Check sheet for the modelled part. Datum: model origin and axes. Units: mm. A direction names the side the tool comes from. Give positions to 0.01 mm unless a question says otherwise; leave off trailing zeros. Order: outer loops, then holes, each group sorted by start corner. A loop starts at its lowest first (then second) coordinate and runs counter-clockwise, first axis right, second up.
```python
from build123d import *

# Parameters (mm, degrees)
EXTRUDE_THIN1_DEPTH = 5
SKETCH2_R           = 2
CUT_EXTRUDE1_DEPTH  = 3
FILLET1_R           = 5
FILLET2_R           = 3
FILLET3_R           = 3
FILLET5_R           = 5


with BuildPart() as part:
    # Sketch1 → Extrude-Thin1 (new body)
    with BuildSketch(Plane.XY):
        with BuildLine():
            ThreePointArc((0, 0), (1.709468812, -15.258106238), (6, -30))
            Line((6, -30), (30, -30))
            Line((30, -30), (30, -40))
            Line((30, -40), (-0.59396654, -40))
            ThreePointArc((-0.59396654, -40), (-7.355075067, -20.616040357), (-9.996685535, -0.257445757))
            Line((-9.996685535, -0.257445757), (0, 0))
        make_face()
    extrude(amount=EXTRUDE_THIN1_DEPTH)

    # Sketch2 → Cut-Extrude1 (cut)
    with BuildSketch(Plane(origin=(0, 0, 0), x_dir=(1, 0, 0), z_dir=(0, 1, 0))):
        with Locations(Location((-4.998342767, -2.5, 0), (0, 0, 270))):
            Circle(SKETCH2_R)
    extrude(amount=-CUT_EXTRUDE1_DEPTH, mode=Mode.SUBTRACT)

    # Fillet1
    fillet1_edges = [part.edges().sort_by_distance(p)[0] for p in [
        (30, -30, 2.5),
    ]]
    fillet(fillet1_edges, radius=FILLET1_R)

    # Fillet2
    fillet2_edges = [part.edges().sort_by_distance(p)[0] for p in [
        (30, -40, 2.5),
    ]]
    fillet(fillet2_edges, radius=FILLET2_R)

    # Fillet3
    fillet3_edges = [part.edges().sort_by_distance(p)[0] for p in [
        (6, -30, 2.5),
    ]]
    fillet(fillet3_edges, radius=FILLET3_R)

    # Fillet4
    # a fillet whose section is not a circle: 5, 0.4 mm, written as the material it takes off along each edge (its section moved 0.00015 mm through the faces so that the kernel can cut it)
    with BuildSketch(Plane(origin=(-22.492542459, -0.579252954, 0), x_dir=(0.02574457573397758, -0.9996685530315923, -2.999999998649999e-05), z_dir=(0.9996685534814432, 0.025744575745562638, 0))) as fillet4_piece_1:
        with BuildLine():
            Bezier((5.000000002, 0), (-0.000149995, 0.000150004), (-0.000162, -0.399999995), weights=[1, 0.707106781, 1])
            Line((-0.000162, -0.399999995), (-0.100162, -0.399996995))
            ThreePointArc((-0.100162, -0.399996995), (-0.100006, -0.199997), (-0.1, 3e-06))
            Line((-0.1, 3e-06), (3e-06, 0.1))
            ThreePointArc((3e-06, 0.1), (2.500002999, 0.099925), (5.000003002, 0.1))
            Line((5.000003002, 0.1), (5.000000002, 0))
        make_face()
    extrude(amount=35.000000011, mode=Mode.SUBTRACT)
    with BuildSketch(Plane(origin=(-9.996685535, -0.257445757, -12.554427483), x_dir=(0.9996611732267645, 0.026029574389313356, 0), z_dir=(0, 0, 1))) as fillet4_piece_2:
        with BuildLine():
            Bezier((0.526141916, 0), (-0.126969786, 0.000186198), (0.12506971, -5.02021329), weights=[1, 0.689048379, 1])
            Line((0.12506971, -5.02021329), (0.02519549, -5.025227283))
            ThreePointArc((0.02519549, -5.025227283), (-0.069016975, -2.513387959), (-0.099999996, 2.8509e-05))
            Line((-0.099999996, 2.8509e-05), (2.8509e-05, 0.099999996))
            ThreePointArc((2.8509e-05, 0.099999996), (0.263099446, 0.099924996), (0.526170426, 0.099999996))
            Line((0.526170426, 0.099999996), (0.526141916, 0))
        make_face()
    extrude(amount=30.108854967, mode=Mode.SUBTRACT)
    with BuildSketch(Plane(origin=(-22.492542459, -0.579252954, 5), x_dir=(-9.654215225776052e-06, 0.00037487568119717526, -0.9999999296875075), z_dir=(0.9996685534814432, 0.025744575745562638, 0))) as fillet4_piece_3:
        with BuildLine():
            Bezier((0.400000028, 0), (-0.000149944, 0.000150056), (-0.002025, -4.999999592), weights=[1, 0.707106781, 1])
            Line((-0.002025, -4.999999592), (-0.102024993, -4.999962092))
            ThreePointArc((-0.102024993, -4.999962092), (-0.100937493, -2.499962324), (-0.099999993, 3.75e-05))
            Line((-0.099999993, 3.75e-05), (3.75e-05, 0.099999993))
            ThreePointArc((3.75e-05, 0.099999993), (0.200037486, 0.099924993), (0.400037528, 0.099999993))
            Line((0.400037528, 0.099999993), (0.400000028, 0))
        make_face()
    extrude(amount=35.000000011, mode=Mode.SUBTRACT)
    with BuildSketch(Plane(origin=(0, 0, -12.449220075), x_dir=(0.05355702462204362, -0.9985647926467435, 0), z_dir=(0, 0, 1))) as fillet4_piece_4:
        with BuildLine():
            Bezier((4.97968803, 0), (-0.004005059, -0.138457778), (-0.00741229, -0.260833255), weights=[1, 0.72649212, 1])
            Line((-0.00741229, -0.260833255), (-0.107373553, -0.25805009))
            ThreePointArc((-0.107373553, -0.25805009), (-0.103592437, -0.12763555), (-0.099961262, 0.002783165))
            Line((-0.099961262, 0.002783165), (0.002783165, 0.099961262))
            ThreePointArc((0.002783165, 0.099961262), (2.489845983, 0.065307551), (4.976910885, 0.09996143))
            Line((4.976910885, 0.09996143), (4.97968803, 0))
        make_face()
    extrude(amount=29.898440151, mode=Mode.SUBTRACT)

    # Fillet5
    fillet5_edges = [part.edges().sort_by_distance(p)[0] for p in [
        (-0.59396654, -40, 2.5),
    ]]
    fillet(fillet5_edges, radius=FILLET5_R)


solid = part.part
```
(1) Release check for a two-part mould opening along Z. For faces 3 (the face through (6, -30, 0)), 4 (the face through (-6.95, -1.51, 2.07)), 5 (the face through (16, -30, 2)) record: released by +Z, released by -Z, zero draft, split by the parting line, or undercut.
Response values:
face 3: released by -Z
face 4: undercut
face 5: zero draft
(2) Cross-section at B-B on y = -29.5. Enter the section's corners in (x, z), then the cut area to 3 significant figures.
Response values:
outline: (-4.81, 0) - (6.42, 0) - (6.42, 5) - (-4.81, 5) - close
area: 56.2 mm2
(3) Gauge pin test, flat ends, axial feed: pin 1 Ø6 at (x, y) = (5.5, -25) entering from +Z; pin 2 Ø3 at (y, z) = (-22, 4) entering from +X. Record the tip position at first contact, or that the pin passes through.
Response values:
pin 1: stops at z = 5
pin 2: stops at x = 3.77
(4) Cross-section at A-A on x = 21. Enter the section's corners in (y, z).
Response values:
outline: (-40, 0) - (-30, 0) - (-30, 5) - (-40, 5) - close
(5) Set-up check for faces 1 (the face through (1.95, -16.43, 2.47)), 2 (the face through (-5, -3, 2)): record each of +Z, -Z, +X, -X, +Y, -Y from which the full face is reachable in a straight line by a thin tool's end or side.
Response values:
face 1: +Z, -Z, +X, +Y
face 2: +Y
(6) Material ranges on L1, parallel to Y at x = 19.5, z = 4.1; L2, parallel to X at y = -1.6, z = 2.5; L3, parallel to X at y = -1.35, z = 2.5, recorded low to high.
Response values:
L1: y = -40 to -30
L2: x = -9.81 to -7, -3 to -0.04
L3: x = -9.79 to -7, -3 to -0.07
